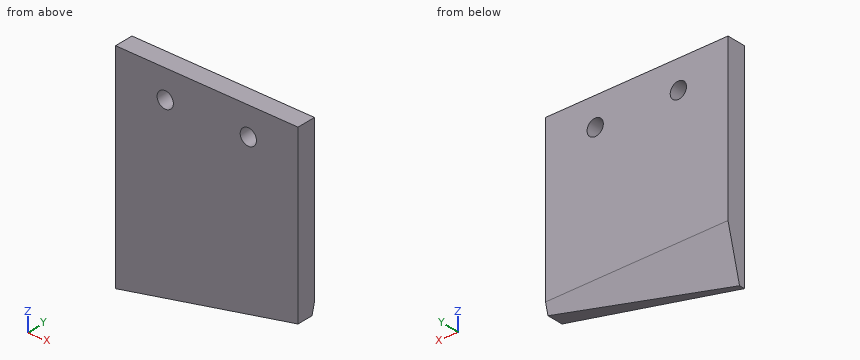
```python
from build123d import *

# Parameters (mm, degrees)
F1_DEPTH = 6.35
F2_R     = 2.73685
F3_DEPTH = 6.35
F5_DEPTH = 63.5


with BuildPart() as f1:
    # F0 (on Front) → F1 (new body)
    with BuildSketch(Plane.XZ):
        Polygon((61.3537, 0), (0, 0), (0, -71.7804), (61.3537, -58.166), align=None)
    extrude(amount=F1_DEPTH)

    # F2 (on face) → F3 (cut)
    with BuildSketch(Plane.XZ.offset(6.35)):
        with Locations((44.64685, -9.46785)):
            Circle(F2_R)
        with Locations((16.70685, -9.46785)):
            Circle(F2_R)
    extrude(amount=-F3_DEPTH, mode=Mode.SUBTRACT)

    # F4 (on face) → F5 (cut)
    with BuildSketch(Plane(origin=(0, 0, 0), x_dir=(0, -1, 0), z_dir=(-1, 0, 0))):
        Polygon((4.45231, -71.7804), (0, -54.5084), (0, -71.7804), align=None)
    extrude(amount=-F5_DEPTH, mode=Mode.SUBTRACT)


solid = f1.part
```
For this review, take the finished solid that the model builds, in its own axes (mm). Round coordinates to 2 decimals unless told otherwise and drop trailing zeros. Loops run counter-clockwise (first coordinate to the right, second up) from the corner with the lowest first, then second, coordinate; pieces in that order, holes last.
(1) Wall thickness on line 1 along Z through (x, y) = (53, -5.25); line 2 along Y through (x, z) = (3, -63); line 3 along Z through (x, y) = (13, -4): over which ranges is each line inside the solid? List them lowest first.
Returned:
line 1: z = -60.02 to 0
line 2: y = -6.35 to -2.19
line 3: z = -68.9 to 0
(2) Clearance check with flat-ended pins moving along their axes: P1, Ø3, axis at x = 11.5, y = -4.5, coming from the +Z side; P2, Ø1, axis at x = 39, y = -3.5, coming from the -Z side; P3, Ø5, axis at x = 44.65, z = -9.47, coming from the +Y side. State where each tip first meets the part, or that it passes through.
Returned:
P1: stops at z = 0
P2: stops at z = -63.24
P3: passes through
(3) We need section A-A (x = 17.5). Give the boundary of the cut face in (y, z), plus the area to 3 significant figures.
Returned:
outline: (-6.35, -67.9) - (-3.45, -67.9) - (0, -54.51) - (0, -12.09) - (-6.35, -12.09) - close; (-6.35, -6.85) - (0, -6.85) - (0, 0) - (-6.35, 0) - close
area: 375 mm2
(4) We need section B-B (y = -2.25). Give the boundary of the cut face in (x, z).
Returned:
outline: (0, -63.24) - (38.5, -63.24) - (61.35, -58.17) - (61.35, 0) - (0, 0) - close; hole circle Ø5.47 at (16.71, -9.47); hole circle Ø5.47 at (44.65, -9.47)
(5) We need section D-D (x = 52). Give the boundary of the cut face in (y, z), plus the area to 3 significant figures.
Returned:
outline: (-6.35, -60.24) - (-1.48, -60.24) - (0, -54.51) - (0, 0) - (-6.35, 0) - close
area: 378 mm2
(6) We need section C-C (z = -8). Give the boundary of the cut face in (x, y), plus the area to 3 significant figures.
Returned:
outline: (0, -6.35) - (14.4, -6.35) - (14.4, 0) - (0, 0) - close; (19.02, -6.35) - (42.34, -6.35) - (42.34, 0) - (19.02, 0) - close; (46.96, -6.35) - (61.35, -6.35) - (61.35, 0) - (46.96, 0) - close
area: 331 mm2
